from build123d import *

# Parameters (mm, degrees)
SKETCH5_R           = 3.175
BOSS_EXTRUDE3_DEPTH = 38.1
CHAMFER1_SIZE       = 0.9525
BOSS_EXTRUDE4_DEPTH = 3.96875
SKETCH8_OUTSIDE_W   = 171.38
SKETCH8_OUTSIDE_H   = 173.1
SKETCH8_OUTSIDE_R   = 5.55625
CUT_EXTRUDE3_DEPTH  = 43.06875
CUT_EXTRUDE3_TAPER  = 60
CUT_EXTRUDE4_DEPTH  = 0.254
CIRPATTERN1_COUNT   = 3


with BuildPart() as part:
    # Sketch5 → Boss-Extrude3 (new body)
    with BuildSketch(Plane(origin=(21.034375, 0, 0), x_dir=(0, 0, -1), z_dir=(1, 0, 0))):
        Circle(SKETCH5_R)
    extrude(amount=-BOSS_EXTRUDE3_DEPTH)

    # Chamfer1
    chamfer1_edges = [part.edges().sort_by_distance(p)[0] for p in [
        (21.034375, 0, 3.175),
    ]]
    chamfer(chamfer1_edges, length=CHAMFER1_SIZE)

    # Sketch11 → Revolve1 (revolve)
    with BuildSketch(Plane.XY):
        Polygon((-17.065625, 3.175), (-17.065625, 0), (5.159375, 0), (1.984375, 3.175), align=None)
    revolve(axis=Axis((-17.065625, 0, 0), (1, 0, 0)))

    # Sketch6 → Boss-Extrude4 (add)
    with BuildSketch(Plane.ZY.offset(17.065625)):
        Polygon((5.55625, 3.207902433), (0, 6.415804866), (-5.55625, 3.207902433), (-5.55625, -3.207902433), (0, -6.415804866), (5.55625, -3.207902433), align=None)
    extrude(amount=BOSS_EXTRUDE4_DEPTH)

    # Sketch8 outside → Cut-Extrude3 (cut, through all)
    with BuildSketch(Plane.ZY.offset(21.034375)):
        Rectangle(SKETCH8_OUTSIDE_W, SKETCH8_OUTSIDE_H)
        Circle(SKETCH8_OUTSIDE_R, mode=Mode.SUBTRACT)
    extrude(amount=-CUT_EXTRUDE3_DEPTH, taper=CUT_EXTRUDE3_TAPER, mode=Mode.SUBTRACT)

    # Sketch12 → Cut-Extrude4 (cut)
    with BuildSketch(Plane.ZY.offset(21.034375)):
        with BuildLine():
            Line((0.1666875, 4.2783125), (0.1666875, 2.3891875))
            ThreePointArc((0.1666875, 2.3891875), (0, 2.2225), (-0.1666875, 2.3891875))
            Line((-0.1666875, 2.3891875), (-0.1666875, 4.2783125))
            ThreePointArc((-0.1666875, 4.2783125), (0, 4.445), (0.1666875, 4.2783125))
        make_face()
    cut_extrude4 = extrude(amount=-CUT_EXTRUDE4_DEPTH, mode=Mode.SUBTRACT)

    # CirPattern1: Cut-Extrude4 ×3 about axis
    cirpattern1_axis = Axis((0, 0, 0), (1, 0, 0))
    for i in range(1, CIRPATTERN1_COUNT):
        add(cut_extrude4.rotate(cirpattern1_axis, i * 360 / CIRPATTERN1_COUNT), mode=Mode.SUBTRACT)


solid = part.part
Input: part model. Units: mm. Frame: model coordinates. A direction names the side the tool comes from. Coordinates: 2 decimals unless noted, no trailing zeros. Loops run counter-clockwise (first coordinate to the right, second up) from the corner with the lowest first, then second, coordinate; pieces in that order, holes last.
Q1. Cut plane A-A (x = -17.5). Output: boundary loops of the cut face in (y, z).
Q2. Material intervals for line 1 (X direction, y = 3, z = -4.25); line 2 (Y direction, x = -0.5, z = 0) (3 decimals); line 3 (X direction, y = -6, z = -0.5), sorted ascending.
Q3. Contact query for flat-ended pins moving along their axis: pin 1 (4 mm diameter, centred on x = -10.5, y = -2.5, fed in from +Z); pin 2 (1.5 mm diameter, centred on x = -14, y = 3.5, fed in from -Z); pin 3 (1 mm diameter, centred on x = -16.5, z = -3, fed in from -Y); pin 4 (1.4 mm diameter, centred on y = -1.5, z = 2.5, fed in from -X). Output: stop coordinate, or through.
Q4. Set-up query: faces 1 (the face through (-20.78, -1.68, 2.9)), 2 (the face through (-19, 0, -5.556)), 3 (the face through (-17.066, -3, -3)). Return all of +Z, -Z, +X, -X, +Y, -Y with unobstructed straight access to the full face (end or side cutting, diameter ignored); none if empty.
Q5. Cut plane B-B (x = -4). Output: boundary loops of the cut face in (y, z) (3 decimals), then the cut area to 3 significant figures.
Q6. Draft query along Z for faces 4 (the face through (-20.78, -1.67, -2.9)), 5 (the face through (-19, 0, 5.556)), 6 (the face through (21.034, 0, 0)). Return one class per face: +Z half, -Z half, draft (parallel to the pull), parting line (faces both ways), or undercut.
Working result:
1. outline: (-6.42, 0) - (-3.21, -5.56) - (3.21, -5.56) - (6.42, 0) - (3.21, 5.56) - (-3.21, 5.56) - close
2. line 1: x = -21.03 to -17.07
2. line 2: y = -3.175 to 3.175
2. line 3: x = -20.77 to -17.07
3. pin 1: stops at z = 3.14
3. pin 2: stops at z = -1.59
3. pin 3: stops at y = -1.96
3. pin 4: stops at x = -21.03
4. face 1: -X
4. face 2: -Z, +X, -X, +Y, -Y
4. face 3: +X
5. outline: circle Ø6.35 at (0, 0)
5. area: 31.7 mm2
6. face 4: undercut
6. face 5: +Z half
6. face 6: draft
